Source: CAD feature listing. Evaluate the final solid. Frame: model axes, mm. Round coordinates to 2 decimals unless told otherwise and drop trailing zeros. Write each loop counter-clockwise with the first axis right and the second up, starting at its lowest first coordinate (ties: lowest second). Pieces come first, ordered by that corner, then holes. Notation, with made-up numbers: (40.5, -15) -> (47.5, -15) arc R29 ccw to (47.5, 24) -> close; hole circle Ø3 at (49, 31.5). An arc over 180 degrees is marked (long way). Put each result on its own line as item: value.
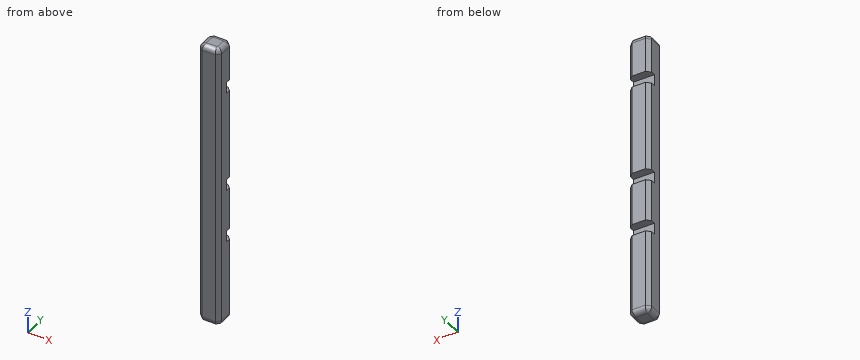
```python
from build123d import *

# Parameters (mm, degrees)
SKETCH1_W           = 8.3
SKETCH1_H           = 8
BOSS_EXTRUDE1_DEPTH = 113.5
CHAMFER2_SIZE       = 1.5
SKETCH3_W           = 8.3
SKETCH3_H           = 3.25
CUT_EXTRUDE1_DEPTH  = 4.5
SKETCH4_W           = 8.3
SKETCH4_H           = 3.25
CUT_EXTRUDE2_DEPTH  = 4.5
FILLET1_R           = 2
SKETCH6_W           = 8.3
SKETCH6_H           = 3.25
CUT_EXTRUDE3_DEPTH  = 4.5


with BuildPart() as part:
    # Sketch1 → Boss-Extrude1 (new body)
    with BuildSketch(Plane.XY):
        Rectangle(SKETCH1_W, SKETCH1_H)
    extrude(amount=BOSS_EXTRUDE1_DEPTH)

    # Chamfer2
    chamfer2_edges = [part.edges().sort_by_distance(p)[0] for p in [
        (-4.15, 4, 56.75),
        (4.15, 4, 56.75),
        (4.15, -4, 56.75),
        (-4.15, -4, 56.75),
    ]]
    chamfer(chamfer2_edges, length=CHAMFER2_SIZE)

    # Sketch3 → Cut-Extrude1 (cut)
    with BuildSketch(Plane(origin=(0, 0, 58), x_dir=(-1, 0, 0), z_dir=(0, 0, -1))):
        with Locations((0, 2.375)):
            Rectangle(SKETCH3_W, SKETCH3_H)
    extrude(amount=CUT_EXTRUDE1_DEPTH, mode=Mode.SUBTRACT)

    # Sketch4 → Cut-Extrude2 (cut)
    with BuildSketch(Plane(origin=(0, 0, 98), x_dir=(-1, 0, 0), z_dir=(0, 0, -1))):
        with Locations((0, 2.375)):
            Rectangle(SKETCH4_W, SKETCH4_H)
    extrude(amount=CUT_EXTRUDE2_DEPTH, mode=Mode.SUBTRACT)

    # Fillet1
    fillet1_edges = [part.edges().sort_by_distance(p)[0] for p in [
        (4.15, 0, 0),
        (4.15, 0, 113.5),
        (-4.15, 0, 0),
        (0, 4, 0),
        (0, -4, 0),
        (-3.4, 3.25, 0),
        (3.4, 3.25, 0),
        (-3.4, -3.25, 0),
        (3.4, -3.25, 0),
        (0, -4, 113.5),
        (-4.15, 0, 113.5),
        (0, 4, 113.5),
        (-3.4, 3.25, 113.5),
        (3.4, 3.25, 113.5),
        (-3.4, -3.25, 113.5),
        (3.4, -3.25, 113.5),
    ]]
    fillet(fillet1_edges, radius=FILLET1_R)

    # Sketch6 → Cut-Extrude3 (cut)
    with BuildSketch(Plane(origin=(0, 0, 37), x_dir=(-1, 0, 0), z_dir=(0, 0, -1))):
        with Locations((0, 2.375)):
            Rectangle(SKETCH6_W, SKETCH6_H)
    extrude(amount=CUT_EXTRUDE3_DEPTH, mode=Mode.SUBTRACT)


solid = part.part
```
Q1. Material intervals for line 1 (Z direction, x = -2.25, y = 1.25); line 2 (Z direction, x = 2.25, y = 3.5); line 3 (Z direction, x = -2.25, y = -1.25), sorted ascending. Write a range as [from, to].
Ans:
line 1: z = [0, 32.5], [37, 53.5], [58, 93.5], [98, 113.5]
line 2: z = [0.68, 32.5], [37, 53.5], [58, 93.5], [98, 112.82]
line 3: z = [0, 113.5]
Q2. Pin query (flat end, axial travel): pin 1 (1.3 mm diameter, centred on x = 1.5, z = 55.5, fed in from +Y); pin 2 (1 mm diameter, centred on x = -0.5, y = 3, fed in from -Z). Return the tip coordinate at first contact, or that it passes through.
Ans:
pin 1: stops at y = 0.75
pin 2: stops at z = 0.06
Q3. Cut plane A-A on x = 0.25. Output: boundary loops of the cut face in (y, z).
Ans:
outline: (-4, 2) arc R2 ccw to (-2, 0) -> (2, 0) arc R2 ccw to (4, 2) -> (4, 32.5) -> (0.75, 32.5) -> (0.75, 37) -> (4, 37) -> (4, 53.5) -> (0.75, 53.5) -> (0.75, 58) -> (4, 58) -> (4, 93.5) -> (0.75, 93.5) -> (0.75, 98) -> (4, 98) -> (4, 111.5) arc R2 ccw to (2, 113.5) -> (-2, 113.5) arc R2 ccw to (-4, 111.5) -> close
Q4. Cut plane B-B on z = 51. Output: boundary loops of the cut face in (x, y), and give its area (3 significant figures).
Ans:
outline: (-4.15, -2.5) -> (-2.65, -4) -> (2.65, -4) -> (4.15, -2.5) -> (4.15, 2.5) -> (2.65, 4) -> (-2.65, 4) -> (-4.15, 2.5) -> close
area: 61.9 mm^2
